```python
from build123d import *

# Parameters (mm, degrees)
SKETCH_1_R               = 27.5
SKETCH_1_R_2             = 17.5
EXTRUDE_1_DEPTH          = 5
SKETCH_2_R               = 27.5
SKETCH_2_R_2             = 18.5
EXTRUDE_2_DEPTH          = 5
EXTRUDE_3_DEPTH          = 9
SKETCH_7_R               = 18.5
CUT_EXTRUDE_4_DEPTH      = 4
SKETCH_13_R              = 9.5
CUT_EXTRUDE_9_DEPTH      = 7
SKETCH_14_R              = 8.5
CUT_EXTRUDE_10_DEPTH     = 3
SKETCH_26_W              = 65.286774434
SKETCH_26_H              = 14.284249769
CUT_EXTRUDE_11_DEPTH     = 1111
SKETCH_28_R              = 18.5
SKETCH_28_R_2            = 17.5
EXTRUDE_4_DEPTH          = 1
HOLE_WIZARD_M3_1_D       = 2.5
PATTERN_CIRCULAR_1_COUNT = 6
HOLE_WIZARD_M3_2_D       = 2.5
PATTERN_CIRCULAR_2_COUNT = 6


with BuildPart() as part:
    # 스케치1 → 보스-돌출1 (new body)
    with BuildSketch(Plane(origin=(0, 0, 0), x_dir=(1, 0, 0), z_dir=(0, 1, 0))):
        Circle(SKETCH_1_R)
        Circle(SKETCH_1_R_2, mode=Mode.SUBTRACT)
    extrude(amount=EXTRUDE_1_DEPTH)

    # 스케치2 → 보스-돌출2 (add)
    with BuildSketch(Plane(origin=(0, 5, 0), x_dir=(1, 0, 0), z_dir=(0, 1, 0))):
        Circle(SKETCH_2_R)
        Circle(SKETCH_2_R_2, mode=Mode.SUBTRACT)
    extrude(amount=EXTRUDE_2_DEPTH)

    # 스케치3 → 보스-돌출3 (add)
    with BuildSketch(Plane(origin=(0, 10, 0), x_dir=(1, 0, 0), z_dir=(0, 1, 0))):
        with BuildLine():
            Line((4.125, 27.188864908), (62.775, 18.290690938))
            ThreePointArc((62.775, 18.290690938), (78.5, 0), (62.775, -18.290690938))
            Line((62.775, -18.290690938), (4.125, -27.188864908))
            ThreePointArc((4.125, -27.188864908), (27.5, 0), (4.125, 27.188864908))
        make_face()
    extrude(amount=-EXTRUDE_3_DEPTH)

    # 스케치7 → 컷-돌출4 (cut)
    with BuildSketch(Plane(origin=(0, 5, 0), x_dir=(1, 0, 0), z_dir=(0, 1, 0))):
        Circle(SKETCH_7_R)
    extrude(amount=-CUT_EXTRUDE_4_DEPTH, mode=Mode.SUBTRACT)

    # 스케치13 → 컷-돌출9 (cut)
    with BuildSketch(Plane.XZ.offset(-1)):
        with Locations((60, 0)):
            Circle(SKETCH_13_R)
    extrude(amount=-CUT_EXTRUDE_9_DEPTH, mode=Mode.SUBTRACT)

    # 스케치14 → 컷-돌출10 (cut, through all)
    with BuildSketch(Plane.XZ.offset(-8)):
        with Locations((60, 0)):
            Circle(SKETCH_14_R)
    extrude(amount=-CUT_EXTRUDE_10_DEPTH, mode=Mode.SUBTRACT)

    # 스케치26 → 컷-돌출11 (cut, symmetric)
    with BuildSketch(Plane(origin=(0, 0, 0), x_dir=(0, 0, -1), z_dir=(1, 0, 0))):
        with Locations((-1.179133759, -1.142124885)):
            Rectangle(SKETCH_26_W, SKETCH_26_H)
    extrude(amount=CUT_EXTRUDE_11_DEPTH, both=True, mode=Mode.SUBTRACT)

    # 스케치28 → 보스-돌출4 (add)
    with BuildSketch(Plane(origin=(0, 10, 0), x_dir=(1, 0, 0), z_dir=(0, 1, 0))):
        Circle(SKETCH_28_R)
        Circle(SKETCH_28_R_2, mode=Mode.SUBTRACT)
    extrude(amount=-EXTRUDE_4_DEPTH)

    # M3 탭을 위한 탭 드릴1 (through all)
    with Locations(Plane(origin=(0, 6, 0), x_dir=(-1, 0, 0), z_dir=(0, -1, 0))):
        with Locations((0, 22.5)):
            hole_wizard_m3_1 = Hole(HOLE_WIZARD_M3_1_D / 2)

    # 원형 패턴1: M3 탭을 위한 탭 드릴1 ×6 about axis
    pattern_circular_1_axis = Axis((0, 0, 0), (0, 1, 0))
    for i in range(1, PATTERN_CIRCULAR_1_COUNT):
        add(hole_wizard_m3_1.rotate(pattern_circular_1_axis, i * 360 / PATTERN_CIRCULAR_1_COUNT), mode=Mode.SUBTRACT)

    # M3 탭을 위한 탭 드릴2 (through all)
    with Locations(Plane(origin=(0, 6, 0), x_dir=(-1, 0, 0), z_dir=(0, -1, 0))):
        with Locations((-60, 13.5)):
            hole_wizard_m3_2 = Hole(HOLE_WIZARD_M3_2_D / 2)

    # 원형 패턴2: M3 탭을 위한 탭 드릴2 ×6 about axis
    pattern_circular_2_axis = Axis((60, 0, 0), (0, 1, 0))
    for i in range(1, PATTERN_CIRCULAR_2_COUNT):
        add(hole_wizard_m3_2.rotate(pattern_circular_2_axis, i * 360 / PATTERN_CIRCULAR_2_COUNT), mode=Mode.SUBTRACT)


solid = part.part
```
Part model, mm, in its own coordinate system. A direction names the side the tool comes from. Round coordinates to 2 decimals unless told otherwise and drop trailing zeros. Write each loop counter-clockwise with the first axis right and the second up, starting at its lowest first coordinate (ties: lowest second). Pieces come first, ordered by that corner, then holes. Notation, with made-up numbers: (70.25, 34) -> (109.25, 34) arc R22 ccw to (109.25, 44) -> close; hole circle Ø5 at (-12.5, -23). An arc over 180 degrees is marked (long way). Return JSON: item names as keys, results as strings. Group by question number.
Q1. Mould opens along Z. For faces 1 (the cylindrical face through (-27.492, 7.972, -0.663)), 2 (the cylindrical face through (-4.01, 7.48, 18.06)), 3 (the flat face through (26, 6, 0)), 4 (the cylindrical face through (47.116, 8.028, -6.375)) say: pulls with the +Z half, pulls with the -Z half, needs draft (parallel to the pull), parting line crosses it, or undercut.
Q2. Pin check, flat tips, straight feed: pin 1 (3 mm diameter, centred on x = 0, z = -22.5, fed in from +Y); pin 2 (2 mm diameter, centred on y = 9, z = -0.5, fed in from -X); pin 3 (1 mm diameter, centred on x = 7.5, y = 8.5, fed in from +Z); pin 4 (1.5 mm diameter, centred on x = 13.5, y = 9, fed in from -Z). Stop position of each tip, or through.
Q3. Which spindle directions (+Z, -Z, +X, -X, +Y, -Y) get a long thin tool onto all of the face, cutting with end or side? Do faces 5 (the cylindrical face through (69.061, 6.986, 2.854)), 6 (the cylindrical face through (61.19, 8.03, -13.88)). Say none if no direction does.
Q4. Saw through at C-C on x = 53.5. Write the cut outline in (y, z).
Q5. Saw through at B-B on z = -4. Write the cut outline in (x, y).
Q6. Saw through at D-D on z = -22.5. Write the cut outline in (x, y), plus the area to 3 significant figures.
Q7. Probe L1, parallel to X at y = 9.2, z = -10.5; L2, parallel to X at y = 8.5, z = -13.5; L3, parallel to X at y = 8.6, z = 5. List the from-to ranges inside material, lowest first. Write a range as [from, to].
Q8. Saw through at A-A on x = 0. Write the cut outline in (y, z).
Answer:
{
 "1": {"face 1": "parting line crosses it", "face 2": "undercut", "face 3": "needs draft", "face 4": "undercut"},
 "2": {"pin 1": "y = 10", "pin 2": "x = -27.5", "pin 3": "z = 26.75", "pin 4": "z = -25.88"},
 "3": {"face 5": "-Y", "face 6": "+Y, -Y"},
 "4": {"outline": "(6, -19.7) -> (10, -19.7) -> (10, -5.48) -> (8, -5.48) -> (8, -6.93) -> (6, -6.93) -> close; (6, 6.93) -> (8, 6.93) -> (8, 5.48) -> (10, 5.48) -> (10, 19.7) -> (6, 19.7) -> close"},
 "5": {"outline": "(-27.21, 6) -> (-18.06, 6) -> (-18.06, 9) -> (-17.04, 9) -> (-17.04, 10) -> (-27.21, 10) -> close; (17.04, 9) -> (18.06, 9) -> (18.06, 6) -> (51.38, 6) -> (51.38, 8) -> (52.5, 8) -> (52.5, 10) -> (17.04, 10) -> close; (67.5, 8) -> (68.62, 8) -> (68.62, 6) -> (78.06, 6) -> (78.06, 10) -> (67.5, 10) -> close"},
 "6": {"outline": "(-15.81, 6) -> (-1.25, 6) -> (-1.25, 10) -> (-15.81, 10) -> close; (1.25, 6) -> (35.03, 6) -> (35.03, 10) -> (1.25, 10) -> close", "area": "193 mm2"},
 "7": {"L1": "[-25.42, -20.49], [-18.49, -14], [14, 18.49], [20.49, 75.23]", "L2": "[-23.96, -12.65], [12.65, 58.75], [61.25, 72.65]", "L3": "[-27.04, -17.81], [17.81, 53.13], [66.87, 77.81]"},
 "8": {"outline": "(6, -27.5) -> (10, -27.5) -> (10, -23.75) -> (6, -23.75) -> close; (6, -21.25) -> (10, -21.25) -> (10, -17.5) -> (9, -17.5) -> (9, -18.5) -> (6, -18.5) -> close; (6, 18.5) -> (9, 18.5) -> (9, 17.5) -> (10, 17.5) -> (10, 21.25) -> (6, 21.25) -> close; (6, 23.75) -> (10, 23.75) -> (10, 27.5) -> (6, 27.5) -> close"}
}
